```python
from build123d import *

# Parameters (mm, degrees)
SKETCH1_R           = 27.5
SKETCH1_R_2         = 9.55
BOSS_EXTRUDE1_DEPTH = 5
SKETCH2_R           = 3
BOSS_EXTRUDE2_DEPTH = 11.7
BOSS_EXTRUDE3_DEPTH = 11.5
SKETCH6_R           = 27.5
BOSS_EXTRUDE4_DEPTH = 20


with BuildPart() as part:
    # Sketch1 → Boss-Extrude1 (new body)
    with BuildSketch(Plane(origin=(0, 0, 0), x_dir=(1, 0, 0), z_dir=(0, 1, 0))):
        Circle(SKETCH1_R)
        Circle(SKETCH1_R_2, mode=Mode.SUBTRACT)
    extrude(amount=BOSS_EXTRUDE1_DEPTH)

    # Sketch2 → Boss-Extrude2 (add)
    with BuildSketch(Plane(origin=(0, 5, 0), x_dir=(1, 0, 0), z_dir=(0, 1, 0))):
        with Locations((0, 21)):
            Circle(SKETCH2_R)
        with Locations((18.186533479, -10.5)):
            Circle(SKETCH2_R)
        with Locations((-18.186533479, -10.5)):
            Circle(SKETCH2_R)
    extrude(amount=BOSS_EXTRUDE2_DEPTH)

    # Sketch3 → Boss-Extrude3 (add)
    with BuildSketch(Plane(origin=(0, 5, 0), x_dir=(1, 0, 0), z_dir=(0, 1, 0))):
        with BuildLine():
            ThreePointArc((-15.937687574, 22.410714286), (-14.839908311, 15.01860206), (-10.504684652, 8.931379517))
            ThreePointArc((-10.504684652, 8.931379517), (-11.941040775, 6.894163106), (-12.987143879, 4.631634009))
            ThreePointArc((-12.987143879, 4.631634009), (-20.426445069, 5.342436557), (-27.377091675, 2.597085174))
            ThreePointArc((-27.377091675, 2.597085174), (-23.815698604, 13.75), (-15.937687574, 22.410714286))
        make_face()
        with BuildLine():
            ThreePointArc((2.482459227, -13.563013526), (5.586536758, -20.361038617), (11.439404101, -25.007799459))
            ThreePointArc((11.439404101, -25.007799459), (0, -27.5), (-11.439404101, -25.007799459))
            ThreePointArc((-11.439404101, -25.007799459), (-5.586536758, -20.361038617), (-2.482459227, -13.563013526))
            ThreePointArc((-2.482459227, -13.563013526), (0, -13.788326212), (2.482459227, -13.563013526))
        make_face()
        with BuildLine():
            ThreePointArc((10.504684652, 8.931379517), (14.839908311, 15.01860206), (15.937687574, 22.410714286))
            ThreePointArc((15.937687574, 22.410714286), (23.815698604, 13.75), (27.377091675, 2.597085174))
            ThreePointArc((27.377091675, 2.597085174), (20.426445069, 5.342436557), (12.987143879, 4.631634009))
            ThreePointArc((12.987143879, 4.631634009), (11.941040775, 6.894163106), (10.504684652, 8.931379517))
        make_face()
    extrude(amount=BOSS_EXTRUDE3_DEPTH)

    # Sketch6 → Boss-Extrude4 (add)
    with BuildSketch(Plane.XZ):
        Circle(SKETCH6_R)
    extrude(amount=BOSS_EXTRUDE4_DEPTH)


solid = part.part
```
The model under review builds one solid part; all positions refer to its coordinate system, in mm. A direction names the side the tool comes from. Give positions to 0.01 mm unless a question says otherwise; leave off trailing zeros. Write each loop counter-clockwise with the first axis right and the second up, starting at its lowest first coordinate (ties: lowest second). Pieces come first, ordered by that corner, then holes. Notation, with made-up numbers: M 60,-4.75 L 116,-4.75 A17 ccw 116,26.25 Z; hole C 54.25,-27 d8. An arc over 180 degrees is marked long. Write item = value, one per line. Start each with the question number.
Q1. Mouldability with a two-part tool opening along X and no side actions: class faces 1 (the face through (-5.65, 10.67, 20.44)), 2 (the face through (5.522, 10.67, 20.278)), 3 (the face through (0, -20, 0)), 4 (the face through (14.8, 10.67, -14.92)) as released by +X, released by -X, zero draft, split by the parting line, or undercut.
Q2. Clearance check with flat-ended pins moving along their axes: pin 1 (10 mm diameter, centred on x = 12.5, y = -10, fed in from -Z); pin 2 (5 mm diameter, centred on x = -1, y = 0.5, fed in from +Z); pin 3 (11.5 mm diameter, centred on x = 0, z = 0, fed in from +Y). State where each tip first meets the part, or that it passes through.
Q3. For line 1 (X direction, y = 3.5, z = 0); line 2 (Y direction, x = 2, z = -23.5), list the stretches that pass through material, from the lowest coordinate up.
Q4. We need section D-D (y = -15). State the section outline as (x, z) points.
Q5. We need section A-A (y = 6). State the section outline as (x, z) points.
Q6. We need section B-B (z = 0). State the section outline as (x, y) points, plus the area to 3 significant figures.
Q7. Machinability: for faces 5 (the face through (0, 16.5, 22)), 6 (the face through (0, 16.7, -21)), 7 (the face through (15.98, 10.77, 8.47)), which of the approach directions +Z, -Z, +X, -X, +Y, -Y give a long, thin tool a straight path to every point of the face, cutting with its end or side? Answer none if there is none.
Q8. We need section C-C (x = 0). State the section outline as (y, z) points.
Result set:
q1.face_1 = released by -X
q1.face_2 = released by +X
q1.face_3 = zero draft
q1.face_4 = undercut
q2.pin_1 = -26.46
q2.pin_2 = 27.5
q2.pin_3 = 0
q3.line_1 = -27.5 to -9.55, 9.55 to 27.5
q3.line_2 = -20 to 5
q4.outline = C 0,0 d55
q5.outline = M -27.38,-2.6 A27.5 ccw -15.94,-22.41 A16 cw -10.5,-8.93 A13.79 cw -12.99,-4.63 A16 cw Z; C -18.19,10.5 d6; M -11.44,25.01 A16 cw -2.48,13.56 A13.79 cw 2.48,13.56 A16 cw 11.44,25.01 A27.5 ccw Z; C 0,-21 d6; M 10.5,-8.93 A16 cw 15.94,-22.41 A27.5 ccw 27.38,-2.6 A16 cw 12.99,-4.63 A13.79 cw Z; C 18.19,10.5 d6
q6.outline = M -27.5,-20 L 27.5,-20 L 27.5,5 L 9.55,5 L 9.55,0 L -9.55,0 L -9.55,5 L -27.5,5 Z
q6.area = 1,280 mm2
q7.face_5 = +Z, +X, -X, +Y
q7.face_6 = +Z, -Z, +X, -X, +Y
q7.face_7 = +Y
q8.outline = M -20,-27.5 L 5,-27.5 L 5,-24 L 16.7,-24 L 16.7,-18 L 5,-18 L 5,-9.55 L 0,-9.55 L 0,9.55 L 5,9.55 L 5,13.79 L 16.5,13.79 L 16.5,27.5 L -20,27.5 Z
